```python
from build123d import *

# Parameters (mm, degrees)
SKETCH1_W           = 60
SKETCH1_H           = 25
BOSS_EXTRUDE1_DEPTH = 80
SKETCH2_W           = 44
SKETCH2_H           = 8
BOSS_EXTRUDE2_DEPTH = 12
SKETCH3_R           = 1.6
CUT_EXTRUDE1_DEPTH  = 99.510151761
FILLET1_R           = 4
CUT_EXTRUDE2_DEPTH  = 93.522970121
CUT_EXTRUDE3_DEPTH  = 3
SKETCH6_R           = 3.5
CUT_EXTRUDE4_DEPTH  = 3
FILLET2_R           = 3
FILLET3_R           = 3


with BuildPart() as part:
    # Sketch1 → Boss-Extrude1 (new body)
    with BuildSketch(Plane(origin=(0, 0, 0), x_dir=(1, 0, 0), z_dir=(0, 1, 0))):
        Rectangle(SKETCH1_W, SKETCH1_H)
    extrude(amount=BOSS_EXTRUDE1_DEPTH)

    # Sketch2 → Boss-Extrude2 (add)
    with BuildSketch(Plane.XY.offset(12.5)):
        with Locations((0, 6)):
            Rectangle(SKETCH2_W, SKETCH2_H)
        Polygon((-4.5, 48), (-4.5, 54), (-9.5, 54), (-9.5, 42), (-4.5, 42), align=None)
        Polygon((4.5, 48), (4.5, 54), (9.5, 54), (9.5, 42), (4.5, 42), align=None)
    extrude(amount=BOSS_EXTRUDE2_DEPTH)

    # Sketch3 → Cut-Extrude1 (cut, through all)
    with BuildSketch(Plane(origin=(22, 0, 0), x_dir=(0, 0, -1), z_dir=(1, 0, 0))):
        with Locations((-20.5, 6)):
            Circle(SKETCH3_R)
    extrude(amount=-CUT_EXTRUDE1_DEPTH, mode=Mode.SUBTRACT)

    # Fillet1
    fillet1_edges = [part.edges().sort_by_distance(p)[0] for p in [
        (0, 2, 24.5),
        (0, 10, 24.5),
    ]]
    fillet(fillet1_edges, radius=FILLET1_R - 0.0001)  # a hair under: the kernel refuses the full size

    # Sketch4 → Cut-Extrude2 (cut, through all)
    with BuildSketch(Plane(origin=(9.5, 0, 0), x_dir=(0, 0, -1), z_dir=(1, 0, 0))):
        with BuildLine():
            ThreePointArc((-17.25, 48), (-18.02164571, 49.154849416), (-19.383883476, 48.883883476))
            Line((-19.383883476, 48.883883476), (-17.616116524, 47.116116524))
            ThreePointArc((-17.616116524, 47.116116524), (-17.345150584, 47.52164571), (-17.25, 48))
        make_face()
        with BuildLine():
            Line((-17.616116524, 47.116116524), (-19.383883476, 48.883883476))
            ThreePointArc((-19.383883476, 48.883883476), (-19.383883476, 47.116116524), (-17.616116524, 47.116116524))
        make_face()
    extrude(amount=-CUT_EXTRUDE2_DEPTH, mode=Mode.SUBTRACT)

    # Sketch5 → Cut-Extrude3 (cut)
    with BuildSketch(Plane(origin=(9.5, 0, 0), x_dir=(0, 0, -1), z_dir=(1, 0, 0))):
        Polygon((-16.871380461, 45.107175821), (-15.180431003, 47.964013804), (-16.809050541, 50.856837983), (-20.128619539, 50.892824179), (-21.819568997, 48.035986196), (-20.190949459, 45.143162017), align=None)
    extrude(amount=-CUT_EXTRUDE3_DEPTH, mode=Mode.SUBTRACT)

    # Sketch6 → Cut-Extrude4 (cut)
    with BuildSketch(Plane.ZY.offset(9.5)):
        with Locations(Location((18.5, 48, 0), (0, 0, 270))):
            Circle(SKETCH6_R)
    extrude(amount=-CUT_EXTRUDE4_DEPTH, mode=Mode.SUBTRACT)

    # Fillet2
    fillet2_edges = [part.edges().sort_by_distance(p)[0] for p in [
        (-7, 54, 24.5),
        (-7, 42, 24.5),
        (7, 42, 24.5),
        (7, 54, 24.5),
    ]]
    fillet(fillet2_edges, radius=FILLET2_R)

    # Fillet3
    fillet3_edges = [part.edges().sort_by_distance(p)[0] for p in [
        (0, 10, 12.5),
        (-7, 54, 12.5),
        (-7, 42, 12.5),
        (7, 42, 12.5),
        (7, 54, 12.5),
    ]]
    fillet(fillet3_edges, radius=FILLET3_R)


solid = part.part
```
Build history of the part. All positions in model axes, mm. A direction names the side the tool comes from. Give positions to 0.01 mm unless a question says otherwise; leave off trailing zeros. Loops run counter-clockwise (first coordinate to the right, second up) from the corner with the lowest first, then second, coordinate; pieces in that order, holes last. Notation, with made-up numbers: (-3, 50.5) - (3, 50.5) arc R4 cw to (3, 56.5) - close; hole circle Ø7 at (58.25, 59.5). An arc over 180 degrees is marked (long way). Use a Markdown table: item, result.
(1) Band-saw the part on C-C (x = 24). Give the cut face in (y, z).
Taken from the geometry:
| item | result |
|---|---|
| outline | (0, -12.5) - (80, -12.5) - (80, 12.5) - (0, 12.5) - close |
(2) Drop flat-ended pins along their axis: pin 1 Ø3.5 at (y, z) = (49, 19) entering from -X; pin 2 Ø5.5 at (x, z) = (-8, 17) entering from +Y; pin 3 Ø2 at (x, y) = (-16.5, 62) entering from +Z; pin 4 Ø1 at (x, z) = (-5, 4.5) entering from -Y. Give the stop position or say it passes through.
Taken from the geometry:
| item | result |
|---|---|
| pin 1 | x = -6.5 |
| pin 2 | y = 54.27 |
| pin 3 | z = 12.5 |
| pin 4 | y = 0 |
(3) Wall check: line 1 along Y through (x, z) = (-11.5, 20.5); line 2 along Z through (x, y) = (-7.7, 48); line 3 along Y through (x, z) = (-5, 20). Give the ranges that are in metal, low to high.
Taken from the geometry:
| item | result |
|---|---|
| line 1 | 2 to 4.4, 7.6 to 10 |
| line 2 | -12.5 to 15, 22 to 24.5 |
| line 3 | 2 to 4.48, 7.52 to 10, 42 to 54 |
(4) Band-saw the part on D-D (y = 43.5). Give the cut face in (x, z), and give its area (3 significant figures).
Taken from the geometry:
| item | result |
|---|---|
| outline | (-30, -12.5) - (30, -12.5) - (30, 12.5) - (9.5, 12.5) - (9.5, 24.1) - (4.5, 24.1) - (4.5, 12.5) - (-4.5, 12.5) - (-4.5, 24.1) - (-9.5, 24.1) - (-9.5, 12.5) - (-30, 12.5) - close |
| area | 1,620 mm2 |
(5) Band-saw the part on B-B (y = 12). Give the cut face in (x, z), and give its area (3 significant figures).
Taken from the geometry:
| item | result |
|---|---|
| outline | (-30, -12.5) - (30, -12.5) - (30, 12.5) - (22, 12.5) - (22, 12.67) - (-22, 12.67) - (-22, 12.5) - (-30, 12.5) - close |
| area | 1,510 mm2 |
(6) Pull direction Z, two halves, no side cores. Call faces 1 (the face through (0.31, 5.03, 21.77)), 2 (the face through (-7, 42, 18)), 3 (the face through (0, 48, 12.5)): +Z half, -Z half, draft (parallel to the pull), parting line (faces both ways), or undercut.
Taken from the geometry:
| item | result |
|---|---|
| face 1 | undercut |
| face 2 | draft |
| face 3 | +Z half |
(7) Which spindle directions (+Z, -Z, +X, -X, +Y, -Y) get a long thin tool onto all of the face, cutting with end or side? Do faces 4 (the face through (4.5, 48, 17)), 5 (the face through (6.96, 41.1, 13.36)), 6 (the face through (8.021, 49.484, 20.962)), 7 (the face through (-7, 54, 18)), 8 (the face through (-22, 6, 18)). Say none if no direction does.
Taken from the geometry:
| item | result |
|---|---|
| face 4 | +Z, +Y |
| face 5 | +Z, +X, -X |
| face 6 | +X |
| face 7 | +Z, +X, -X, +Y |
| face 8 | +Z, -X, +Y, -Y |
